```python
from build123d import *

# Parameters (mm, degrees)
SKETCH1_W           = 13
SKETCH1_H           = 5
BOSS_EXTRUDE1_DEPTH = 11
SKETCH2_W           = 13
SKETCH2_H           = 3
CUT_EXTRUDE1_DEPTH  = 9
SKETCH3_W           = 3
SKETCH3_H           = 6
CUT_EXTRUDE2_DEPTH  = 2
SKETCH4_R           = 0.85
BOSS_EXTRUDE3_DEPTH = 9


with BuildPart() as part:
    # Sketch1 → Boss-Extrude1 (new body)
    with BuildSketch(Plane(origin=(0, 0, 0), x_dir=(1, 0, 0), z_dir=(0, 1, 0))):
        with Locations((6.5, 2.5)):
            Rectangle(SKETCH1_W, SKETCH1_H)
    extrude(amount=BOSS_EXTRUDE1_DEPTH)

    # Sketch2 → Cut-Extrude1 (cut)
    with BuildSketch(Plane(origin=(0, 11, 0), x_dir=(1, 0, 0), z_dir=(0, 1, 0))):
        with Locations((6.5, 1.5)):
            Rectangle(SKETCH2_W, SKETCH2_H)
    extrude(amount=-CUT_EXTRUDE1_DEPTH, mode=Mode.SUBTRACT)

    # Sketch3 → Cut-Extrude2 (cut)
    with BuildSketch(Plane(origin=(0, 0, -5), x_dir=(-1, 0, 0), z_dir=(0, 0, -1))):
        with Locations((-6.5, 3)):
            Rectangle(SKETCH3_W, SKETCH3_H)
    extrude(amount=-CUT_EXTRUDE2_DEPTH, mode=Mode.SUBTRACT)

    # Sketch4 → Boss-Extrude3 (add)
    with BuildSketch(Plane(origin=(0, 2, 0), x_dir=(1, 0, 0), z_dir=(0, 1, 0))):
        with Locations(Location((10.5, 2, 0), (0, 0, 90))):
            Circle(SKETCH4_R)
        with Locations(Location((6.5, 2, 0), (0, 0, 90))):
            Circle(SKETCH4_R)
        with Locations(Location((2.5, 2, 0), (0, 0, 90))):
            Circle(SKETCH4_R)
    extrude(amount=BOSS_EXTRUDE3_DEPTH)


solid = part.part
```
The model under review builds one solid part; all positions refer to its coordinate system, in mm. A direction names the side the tool comes from. Round coordinates to 2 decimals unless told otherwise and drop trailing zeros. Write each loop counter-clockwise with the first axis right and the second up, starting at its lowest first coordinate (ties: lowest second). Pieces come first, ordered by that corner, then holes.
(1) We need section D-D on y = 5. Give the boundary of the cut face in (x, z).
(2) We need section B-B on x = 6.5. Give the boundary of the cut face in (y, z), and give its area (3 significant figures).
(3) Insertion check: pin 1 (4.5 mm diameter, centred on x = 4, y = 7, fed in from +Z); pin 2 (1 mm diameter, centred on x = 6, y = 1.5, fed in from -Z). Each pin has a flat end and moves straight along its axis. Give the tip position at first contact, or say it passes through.
(4) Wall thickness on L1, parallel to Z at x = 10.5, y = 6.5; L2, parallel to X at y = 4, z = -4.65; L3, parallel to Y at x = 1.25, z = -2.5: over which ranges is each line inside the solid? List them lowest first.
(5) Mouldability with a two-part tool opening along X and no side actions: class faces 1 (the flat face through (6, 11, -2)), 2 (the flat face through (13, 4, -4)), 3 (the flat face through (0, 4, -4)), 4 (the flat face through (6, 2, -1)) as +X half, -X half, draft (parallel to the pull), parting line (faces both ways), or undercut.
(6) We need section A-A on y = 7. Give the boundary of the cut face in (x, z), and give its area (3 significant figures).
(7) Machinability: for faces 5 (the flat face through (10, 11, -2)), 6 (the cylindrical face through (6.24, 6.44, -2.81)), 7 (the flat face through (6, 7, -3)), 8 (the flat face through (8, 3, -4)), which of the approach directions +Z, -Z, +X, -X, +Y, -Y give a long, thin tool a straight path to every point of the face, cutting with its end or side? Answer none if there is none.
(8) We need section C-C on z = -2. Give the boundary of the cut face in (x, y).
Findings below:
1. outline: (0, -5) - (5, -5) - (5, -3) - (0, -3) - close; circle Ø1.7 at (2.5, -2); circle Ø1.7 at (6.5, -2); (8, -5) - (13, -5) - (13, -3) - (8, -3) - close; circle Ø1.7 at (10.5, -2)
2. outline: (0, -3) - (2, -3) - (2, -2.85) - (11, -2.85) - (11, -1.15) - (2, -1.15) - (2, 0) - (0, 0) - close; (6, -5) - (11, -5) - (11, -3) - (6, -3) - close
2. area: 31.3 mm2
3. pin 1: stops at z = -1.15
3. pin 2: stops at z = -3
4. L1: z = -5 to -3, -2.85 to -1.15
4. L2: x = 0 to 5, 8 to 13
4. L3: y = 0 to 2
5. face 1: draft
5. face 2: +X half
5. face 3: -X half
5. face 4: undercut
6. outline: (0, -5) - (13, -5) - (13, -3) - (0, -3) - close; circle Ø1.7 at (2.5, -2); circle Ø1.7 at (6.5, -2); circle Ø1.7 at (10.5, -2)
6. area: 32.8 mm2
7. face 5: +Z, -Z, +X, -X, +Y
7. face 6: +Y
7. face 7: +X, -X, +Y
7. face 8: -Z, -Y
8. outline: (0, 0) - (13, 0) - (13, 2) - (11.35, 2) - (11.35, 11) - (9.65, 11) - (9.65, 2) - (7.35, 2) - (7.35, 11) - (5.65, 11) - (5.65, 2) - (3.35, 2) - (3.35, 11) - (1.65, 11) - (1.65, 2) - (0, 2) - close
